Design review of the part built by this model. Coordinates are the model's own, in mm. Coordinates: 2 decimals unless noted, no trailing zeros. One line per item, written item: value. Start each with the question number.
1. Add section A-A on x = 584. Give the number of separate pieces and of enclosed holes in the cut face, plus the area to 3 significant figures.
2. Insertion check: pin 1 (22 mm diameter, centred on y = -321, z = 23.5, fed in from -X). The pin has a flat end and moves straight along its axis. Give the tip position at first contact, or say it passes through.
3. For probe 1 along Y at (x, z) = (1259, 48.5) (3 decimals); probe 2 along Z at (x, y) = (859.5, -877) (3 decimals); probe 3 along X at (y, z) = (-490, 3), list the stretches that pass through material, from the lowest coordinate up.
```python
from build123d import *

# Parameters (mm, degrees)
F0_W     = 1524
F0_H     = 1066.8
F0_W_2   = 660.4
F0_H_2   = 31.75
F0_W_3   = 304.8
F1_DEPTH = 50.8
F3_R     = 6.35
F4_DEPTH = 127
F5_T     = -3.175


# Not quite as in the source:
# - a feature names something its author has since deleted; it is built from what else it names


with BuildPart() as f1:
    # F0 (on Top) → F1 (new body)
    with BuildSketch(Plane.XY):
        with Locations((762, -533.4)):
            Rectangle(F0_W, F0_H)
        Polygon((1011.4551224214, -1035.05), (831.85, -1035.05), (831.85, -855.4448775786), (831.85, -810.5435969733), (831.85, -581.025), (1492.25, -581.025), (1492.25, -788.03246), (1492.25, -832.48246), (1492.25, -846.4646214575), (1492.25, -891.3659020629), (1492.25, -1035.05), (1348.5659020629, -1035.05), (1303.6646214575, -1035.05), (1056.3564030267, -1035.05), align=None, mode=Mode.SUBTRACT)
        Polygon((31.75, -175.4340979371), (31.75, -31.75), (175.4340979371, -31.75), (220.3353785425, -31.75), (463.55, -31.75), (463.55, -298.45), (463.55, -333.4391527639), (463.55, -733.3608472361), (463.55, -768.35), (463.55, -1035.05), (220.3353785425, -1035.05), (175.4340979371, -1035.05), (31.75, -1035.05), (31.75, -891.3659020629), (31.75, -846.4646214575), (31.75, -832.48246), (31.75, -788.03246), (31.75, -568.3891527639), (31.75, -533.4), (31.75, -498.4108472361), (31.75, -220.3353785425), align=None, mode=Mode.SUBTRACT)
        Polygon((800.1, -1035.05), (495.3, -1035.05), (495.3, -768.35), (495.3, -736.6), (495.3, -330.2), (495.3, -298.45), (495.3, -31.75), (800.1, -31.75), (800.1, -298.45), (800.1, -330.2), (800.1, -736.6), (800.1, -768.35), align=None, mode=Mode.SUBTRACT)
        with Locations((1162.05, -533.4)):
            Rectangle(F0_W_2, F0_H_2, mode=Mode.SUBTRACT)
        Polygon((1348.5659020629, -31.75), (1492.25, -31.75), (1492.25, -175.4340979371), (1492.25, -220.3353785425), (1492.25, -485.775), (831.85, -485.775), (831.85, -256.2564030267), (831.85, -211.3551224214), (831.85, -31.75), (1011.4551224214, -31.75), (1056.3564030267, -31.75), (1303.6646214575, -31.75), align=None, mode=Mode.SUBTRACT)
        Polygon((463.55, -298.45), (31.75, -498.4108472361), (31.75, -533.4), (463.55, -333.4391527639), align=None)
        Polygon((463.55, -733.3608472361), (31.75, -533.4), (31.75, -568.3891527639), (463.55, -768.35), align=None)
        with Locations((647.7, -752.475)):
            Rectangle(F0_W_3, F0_H_2)
        with Locations((647.7, -314.325)):
            Rectangle(F0_W_3, F0_H_2)
        Polygon((831.85, -256.2564030267), (1056.3564030267, -31.75), (1011.4551224214, -31.75), (831.85, -211.3551224214), align=None)
        Polygon((831.85, -810.5435969733), (831.85, -855.4448775786), (1011.4551224214, -1035.05), (1056.3564030267, -1035.05), align=None)
        Polygon((220.3353785425, -31.75), (175.4340979371, -31.75), (31.75, -175.4340979371), (31.75, -220.3353785425), align=None)
        Polygon((220.3353785425, -1035.05), (31.75, -846.4646214575), (31.75, -891.3659020629), (175.4340979371, -1035.05), align=None)
        Polygon((1492.25, -846.4646214575), (1303.6646214575, -1035.05), (1348.5659020629, -1035.05), (1492.25, -891.3659020629), align=None)
        Polygon((1492.25, -220.3353785425), (1492.25, -175.4340979371), (1348.5659020629, -31.75), (1303.6646214575, -31.75), align=None)
    extrude(amount=F1_DEPTH)

    # F3 (on face) → F4 (cut)
    with BuildSketch(Plane(origin=(0, -485.775, 0), x_dir=(-1, 0, 0), z_dir=(0, 1, 0))):
        with Locations((-933.45, 25.4)):
            Circle(F3_R)
    extrude(amount=-F4_DEPTH, mode=Mode.SUBTRACT)

    # F5
    f5_openings = [f1.faces().sort_by_distance(p)[0] for p in [
        (939.8, -565.15, 25.4),
        (939.8, -501.65, 25.4),
    ]]
    offset(amount=F5_T, openings=f5_openings, kind=Kind.INTERSECTION)


solid = f1.part
```
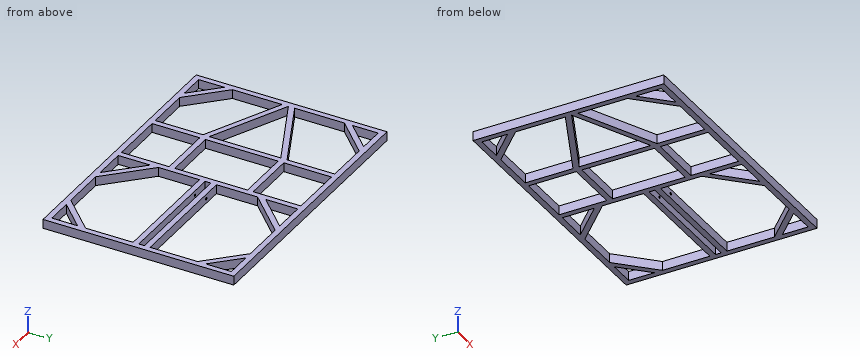
Worked answers:
1. separate pieces: 4
1. enclosed holes: 4
1. area: 1,940 mm²
2. pin 1: stops at x = 0
3. probe 1: y = -1066.8 to -1035.05, -581.025 to -549.275, -517.525 to -485.775, -31.75 to 0
3. probe 2: z = 0 to 3.175, 47.625 to 50.8
3. probe 3: x = 0 to 31.75, 49.91 to 125.47, 463.55 to 495.3, 800.1 to 1524
